```python
from build123d import *

# Parameters (mm, degrees)
SKETCH1_W           = 76.2
SKETCH1_H           = 101.6
SKETCH1_R           = 2.5
BOSS_EXTRUDE1_DEPTH = 6.35
SKETCH2_R           = 2.5781
SKETCH2_R_2         = 1.4351
SKETCH2_R_3         = 2.331256363
SKETCH2_R_4         = 1.188256363
BOSS_EXTRUDE2_DEPTH = 3.175
BOSS_EXTRUDE3_START = 3.175
SKETCH2_4_R         = 1.4351
SKETCH2_4_R_2       = 1.188256363
BOSS_EXTRUDE3_DEPTH = 3.175


with BuildPart() as part:
    # Sketch1 → Boss-Extrude1 (new body)
    with BuildSketch(Plane(origin=(0, 0, 0), x_dir=(1, 0, 0), z_dir=(0, 1, 0))):
        Rectangle(SKETCH1_W, SKETCH1_H)
        with Locations(Location((-31.75, 38.1, 0), (0, 0, 270))):
            Circle(SKETCH1_R, mode=Mode.SUBTRACT)
        with Locations(Location((-31.75, -38.1, 0), (0, 0, 270))):
            Circle(SKETCH1_R, mode=Mode.SUBTRACT)
        with Locations(Location((31.75, 38.1, 0), (0, 0, 270))):
            Circle(SKETCH1_R, mode=Mode.SUBTRACT)
        with Locations(Location((31.75, -38.1, 0), (0, 0, 270))):
            Circle(SKETCH1_R, mode=Mode.SUBTRACT)
    extrude(amount=BOSS_EXTRUDE1_DEPTH)

    # Sketch2 → Boss-Extrude2 (add)
    with BuildSketch(Plane(origin=(0, 6.35, 0), x_dir=(1, 0, 0), z_dir=(0, 1, 0))):
        with Locations(Location((-24.1681, 36.6776, 0), (0, 0, 90))):
            Circle(SKETCH2_R)
        with Locations((-24.1681, 36.6776)):
            Circle(SKETCH2_R_2, mode=Mode.SUBTRACT)
        with Locations((-24.1681, 36.6776)):
            Circle(SKETCH2_R_2)
        with Locations(Location((24.1681, 36.6776, 0), (0, 0, 90))):
            Circle(SKETCH2_R)
        with Locations((24.1681, 36.6776)):
            Circle(SKETCH2_R_2, mode=Mode.SUBTRACT)
        with Locations((24.1681, 36.6776)):
            Circle(SKETCH2_R_2)
        with Locations(Location((-19.289607234, -14.9479, 0), (0, 0, 90))):
            Circle(SKETCH2_R)
        with Locations((-19.289607234, -14.9479)):
            Circle(SKETCH2_R_2, mode=Mode.SUBTRACT)
        with Locations((-19.289607234, -14.9479)):
            Circle(SKETCH2_R_2)
        with Locations(Location((8.726592766, -14.9479, 0), (0, 0, 90))):
            Circle(SKETCH2_R_3)
        with Locations((8.726592766, -14.9479)):
            Circle(SKETCH2_R_4, mode=Mode.SUBTRACT)
        with Locations((8.726592766, -14.9479)):
            Circle(SKETCH2_R_4)
        with Locations(Location((-24.1681, -45.9486, 0), (0, 0, 90))):
            Circle(SKETCH2_R)
        with Locations((-24.1681, -45.9486)):
            Circle(SKETCH2_R_2, mode=Mode.SUBTRACT)
        with Locations((-24.1681, -45.9486)):
            Circle(SKETCH2_R_2)
        with Locations(Location((24.1681, -38.4556, 0), (0, 0, 90))):
            Circle(SKETCH2_R)
        with Locations((24.1681, -38.4556)):
            Circle(SKETCH2_R_2, mode=Mode.SUBTRACT)
        with Locations((24.1681, -38.4556)):
            Circle(SKETCH2_R_2)
    extrude(amount=BOSS_EXTRUDE2_DEPTH)

    # Sketch2<4> → Boss-Extrude3 (add)
    with BuildSketch(Plane(origin=(0, 6.35, 0), x_dir=(1, 0, 0), z_dir=(0, 1, 0)).offset(BOSS_EXTRUDE3_START)):
        with Locations(Location((-24.1681, 36.6776, 0), (0, 0, 270))):
            Circle(SKETCH2_4_R)
        with Locations(Location((24.1681, 36.6776, 0), (0, 0, 270))):
            Circle(SKETCH2_4_R)
        with Locations(Location((-19.289607234, -14.9479, 0), (0, 0, 270))):
            Circle(SKETCH2_4_R)
        with Locations(Location((8.726592766, -14.9479, 0), (0, 0, 270))):
            Circle(SKETCH2_4_R_2)
        with Locations(Location((24.1681, -38.4556, 0), (0, 0, 270))):
            Circle(SKETCH2_4_R)
        with Locations(Location((-24.1681, -45.9486, 0), (0, 0, 270))):
            Circle(SKETCH2_4_R)
    extrude(amount=BOSS_EXTRUDE3_DEPTH)


solid = part.part
```
The model under review builds one solid part; all positions refer to its coordinate system, in mm. A direction names the side the tool comes from. Round coordinates to 2 decimals unless told otherwise and drop trailing zeros. Order: outer loops, then holes, each group sorted by start corner. A loop starts at its lowest first (then second) coordinate and runs counter-clockwise, first axis right, second up. Notation, with made-up numbers: (23.5, 13) - (78.5, 13) arc R32 cw to (78.5, 40) - close; hole circle Ø10 at (33, 87). An arc over 180 degrees is marked (long way). Answer in a Markdown table with one row per item.
(1) Mouldability with a two-part tool opening along Z and no side actions: class faces 1 (the face through (23.62, 11.09, 39.78)), 2 (the face through (-19.227, 11.09, 13.514)), 3 (the face through (10, 9.525, 14)) as released by +Z, released by -Z, zero draft, split by the parting line, or undercut.
Result set:
| item | result |
|---|---|
| face 1 | undercut |
| face 2 | split by the parting line |
| face 3 | zero draft |
(2) Take a section at A-A on x = 31.75. Write out the cut boundary in (y, z).
Result set:
| item | result |
|---|---|
| outline | (0, -50.8) - (6.35, -50.8) - (6.35, -40.6) - (0, -40.6) - close; (0, -35.6) - (6.35, -35.6) - (6.35, 35.6) - (0, 35.6) - close; (0, 40.6) - (6.35, 40.6) - (6.35, 50.8) - (0, 50.8) - close |
(3) Clearance check with flat-ended pins moving along their axes: P1, Ø6.5, axis at x = -31.75, z = 38.1, coming from the +Y side; P2, Ø1.5, axis at x = -29, y = 7.5, coming from the +Z side. State where each tip first meets the part, or that it passes through.
Result set:
| item | result |
|---|---|
| P1 | stops at y = 6.35 |
| P2 | passes through |
(4) For line 1 (X direction, y = 3.5, z = 38.1); line 2 (Z direction, x = 33, y = 4.75); line 3 (Y direction, x = -11, z = -30), list the stretches that pass through material, from the lowest coordinate up. Write a range as from..to.
Result set:
| item | result |
|---|---|
| line 1 | x = -38.1..-34.25, -29.25..29.25, 34.25..38.1 |
| line 2 | z = -50.8..-40.27, -35.93..35.93, 40.27..50.8 |
| line 3 | y = 0..6.35 |
(5) Take a section at B-B on y = 10.75. Write out the cut boundary in (x, z).
Result set:
| item | result |
|---|---|
| outline | circle Ø2.87 at (-24.17, -36.68); circle Ø2.87 at (-24.17, 45.95); circle Ø2.87 at (-19.29, 14.95); circle Ø2.38 at (8.73, 14.95); circle Ø2.87 at (24.17, -36.68); circle Ø2.87 at (24.17, 38.46) |
(6) Take a section at C-C on z = 38.1. Write out the cut boundary in (x, y) (3 decimals).
Result set:
| item | result |
|---|---|
| outline | (-38.1, 0) - (-34.25, 0) - (-34.25, 6.35) - (-38.1, 6.35) - close; (-29.25, 0) - (29.25, 0) - (29.25, 6.35) - (26.722, 6.35) - (26.722, 9.525) - (25.558, 9.525) - (25.558, 12.7) - (22.778, 12.7) - (22.778, 9.525) - (21.615, 9.525) - (21.615, 6.35) - (-29.25, 6.35) - close; (34.25, 0) - (38.1, 0) - (38.1, 6.35) - (34.25, 6.35) - close |
(7) Machinability: for faces 4 (the face through (-24, 9.525, 44)), 5 (the face through (24, 12.7, 38)), which of the approach directions +Z, -Z, +X, -X, +Y, -Y give a long, thin tool a straight path to every point of the face, cutting with its end or side? Answer none if there is none.
Result set:
| item | result |
|---|---|
| face 4 | +Y |
| face 5 | +Z, -Z, +X, -X, +Y |
(8) Take a section at D-D on x = -11.5. Write out the cut boundary in (y, z).
Result set:
| item | result |
|---|---|
| outline | (0, -50.8) - (6.35, -50.8) - (6.35, 50.8) - (0, 50.8) - close |
